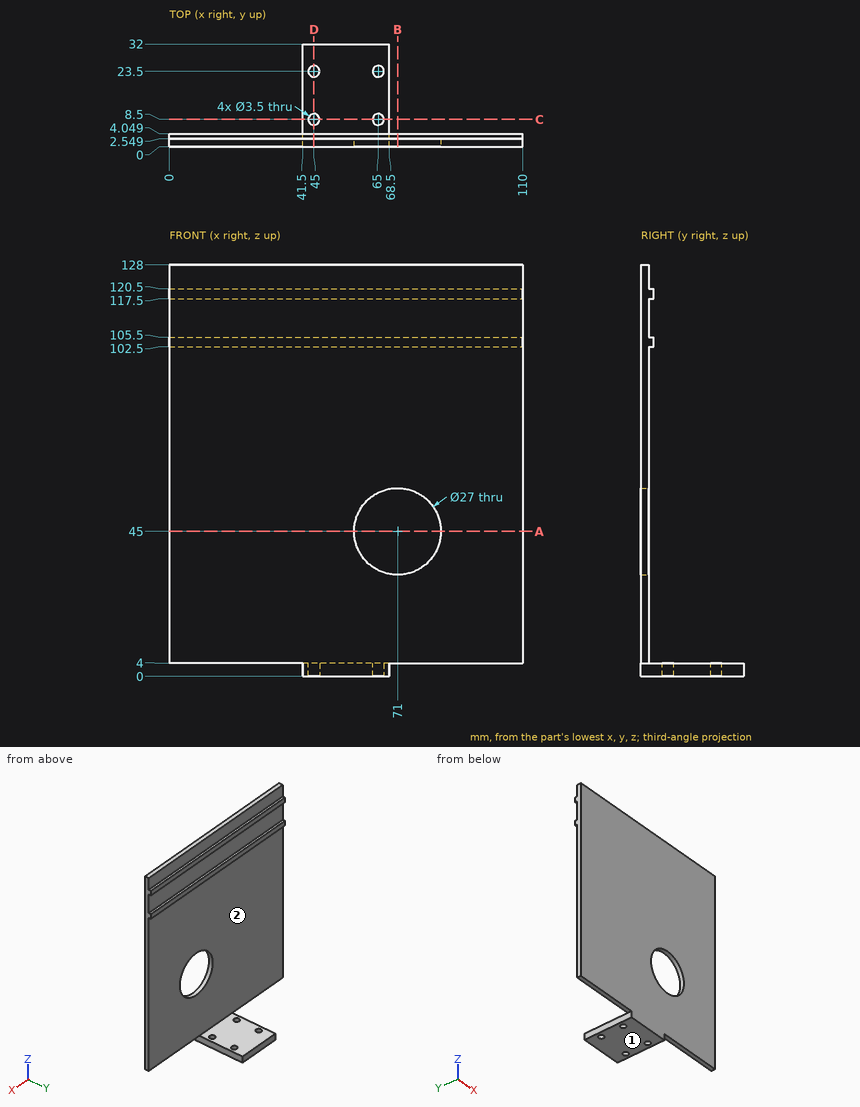
Print and shaded views of the part. All mm, measured from the part's lowest x, y and z. A direction names the side the tool comes from. Coordinates: 2 decimals unless noted, no trailing zeros. Write each loop counter-clockwise with the first axis right and the second up, starting at its lowest first coordinate (ties: lowest second). Pieces come first, ordered by that corner, then holes. Notation, with made-up numbers: (-34, 34) -> (24, 34) arc R26 ccw to (24, 65) -> close; hole circle Ø8 at (64.25, -14). An arc over 180 degrees is marked (long way). Use CSV: the item, a comma, the result in double quotes. Start each with the question number.
Q1. 3-axis set-ups, long thin cutter, end or side, ignore diameter. For the marked faces 1 and 2: which of +Z, -Z, +X, -X, +Y, -Y reach the whole face in a straight line?
Q2. Cut at A-A, the plane z = 45. List the corners of the cut face in (x, y).
Q3. Cut at D-D, the plane x = 45. List the corners of the cut face in (y, z).
Q4. Cut at B-B, the plane x = 71. List the corners of the cut face in (y, z), then the cut area to 3 significant figures.
Q5. Cut at C-C, the plane y = 8.5. List the corners of the cut face in (x, z), then the cut area to 3 significant figures.
Q6. Flat gauge pins, fed straight in: pin 1 Ø1.5 at (x, z) = (61.5, 104) entering from +Y; pin 2 Ø0.5 at (x, y) = (54.5, 3.5) entering from +Z; pin 3 Ø1.3 at (x, y) = (11.5, 1) entering from -Z. Where does each tip first touch, or does it go through?
Q7. Drill centre lines: probe 1 along Y at (x, z) = (65, 2.6); probe 2 along Z at (x, y) = (23.5, 3.5); probe 3 along X at (y, z) = (0.75, 45). Where is each one in solid material? Low to high.
Checked values:
1,face 1,"-Z, +X, -X, +Y, -Y"
1,face 2,"+X, -X, +Y"
2,outline,"(0, 0) -> (57.5, 0) -> (57.5, 2.55) -> (0, 2.55) -> close; (84.5, 0) -> (110, 0) -> (110, 2.55) -> (84.5, 2.55) -> close"
3,outline,"(0, 0) -> (6.75, 0) -> (6.75, 4) -> (2.55, 4) -> (2.55, 102.5) -> (4.05, 102.5) -> (4.05, 105.5) -> (2.55, 105.5) -> (2.55, 117.5) -> (4.05, 117.5) -> (4.05, 120.5) -> (2.55, 120.5) -> (2.55, 128) -> (0, 128) -> close; (10.25, 0) -> (21.75, 0) -> (21.75, 4) -> (10.25, 4) -> close; (25.25, 0) -> (32, 0) -> (32, 4) -> (25.25, 4) -> close"
4,outline,"(0, 4) -> (2.55, 4) -> (2.55, 31.5) -> (0, 31.5) -> close; (0, 58.5) -> (2.55, 58.5) -> (2.55, 102.5) -> (4.05, 102.5) -> (4.05, 105.5) -> (2.55, 105.5) -> (2.55, 117.5) -> (4.05, 117.5) -> (4.05, 120.5) -> (2.55, 120.5) -> (2.55, 128) -> (0, 128) -> close"
4,area,"256 mm²"
5,outline,"(41.5, 0) -> (43.25, 0) -> (43.25, 4) -> (41.5, 4) -> close; (46.75, 0) -> (63.25, 0) -> (63.25, 4) -> (46.75, 4) -> close; (66.75, 0) -> (68.5, 0) -> (68.5, 4) -> (66.75, 4) -> close"
5,area,"80.0 mm²"
6,pin 1,"stops at y = 4.05"
6,pin 2,"stops at z = 120.5"
6,pin 3,"stops at z = 4"
7,probe 1,"y = 0 to 6.75, 10.25 to 21.75, 25.25 to 32"
7,probe 2,"z = 102.5 to 105.5, 117.5 to 120.5"
7,probe 3,"x = 0 to 57.5, 84.5 to 110"
